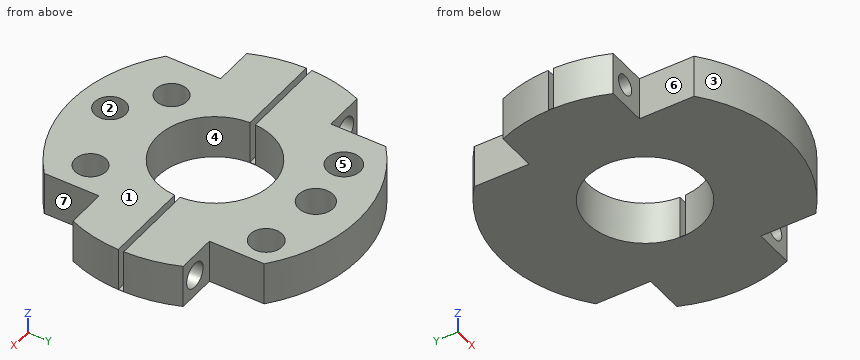
from build123d import *

# Parameters (mm, degrees)
SKETCH_R        = 20
SKETCH_R_2      = 8
PAD_DEPTH       = 6
SKETCH001_R     = 2.4
SKETCH001_R_2   = 2.3
SKETCH001_R_3   = 2.2
SKETCH001_R_4   = 2.15
POCKET_DEPTH    = 4
SKETCH003_W     = 43.022533
SKETCH003_H     = 0.75
POCKET001_DEPTH = 5.95
SKETCH007_W     = 7.6375744751
SKETCH007_H     = 10.86069433
SKETCH007_W_2   = 8.2446434751
SKETCH007_H_2   = 12.05515533
SKETCH007_W_3   = 8.5299164751
SKETCH007_H_3   = 10.94123533
SKETCH007_W_4   = 11.8328734751
SKETCH007_H_4   = 10.66832833
POCKET002_DEPTH = 6.001
SKETCH008_R     = 1.4
POCKET003_DEPTH = 27.65392667
SKETCH009_R     = 1.75
POCKET004_DEPTH = 8


with BuildPart() as part:
    # Sketch → Pad (new body)
    with BuildSketch(Plane.XY):
        Circle(SKETCH_R)
        Circle(SKETCH_R_2, mode=Mode.SUBTRACT)
    extrude(amount=PAD_DEPTH)

    # Sketch001 (on Face4 of Pad) → Pocket (cut)
    with BuildSketch(Plane.XY.offset(6)):
        with Locations((0, 14)):
            Circle(SKETCH001_R)
        with Locations((-7.5, 12.9903810568)):
            Circle(SKETCH001_R_2)
        with Locations((9.1772229816, 13.1064327086)):
            Circle(SKETCH001_R_3)
        with Locations((8.7263178357, -11.5802148957)):
            Circle(SKETCH001_R_4)
        with Locations((-1.3509140126, -15.4410178204)):
            Circle(SKETCH001_R_4)
        with Locations((-7.2695077451, -10.7774884432)):
            Circle(SKETCH001_R_4)
    extrude(amount=-POCKET_DEPTH, mode=Mode.SUBTRACT)

    # Sketch003 (on Face3 of Pocket) → Pocket001 (cut)
    with BuildSketch(Plane.XY.offset(6)):
        with Locations((-0.7364995, 0)):
            Rectangle(SKETCH003_W, SKETCH003_H)
    extrude(amount=-POCKET001_DEPTH, mode=Mode.SUBTRACT)

    # Sketch007 (on Face9 of Pocket001) → Pocket002 (cut, through all)
    with BuildSketch(Plane.XY.offset(6)):
        with Locations((-16.7398847624, -13.083273835)):
            Rectangle(SKETCH007_W, SKETCH007_H)
        with Locations((-17.0434192624, 13.680504335)):
            Rectangle(SKETCH007_W_2, SKETCH007_H_2)
        with Locations((17.1860557624, 13.123544335)):
            Rectangle(SKETCH007_W_3, SKETCH007_H_3)
        with Locations((18.8375342624, -12.987090835)):
            Rectangle(SKETCH007_W_4, SKETCH007_H_4)
    extrude(amount=-POCKET002_DEPTH, mode=Mode.SUBTRACT)

    # Sketch008 → Pocket003 (cut, through all)
    with BuildSketch(Plane(origin=(0, 7.65292667, 0), x_dir=(-1, 0, 0), z_dir=(0, 1, 0))):
        with Locations((-15.963433, 3)):
            Circle(SKETCH008_R)
        with Locations((15.963433, 3)):
            Circle(SKETCH008_R)
    extrude(amount=-POCKET003_DEPTH, mode=Mode.SUBTRACT)

    # Sketch009 → Pocket004 (cut)
    with BuildSketch(Plane(origin=(0, 7.65292667, 0), x_dir=(-1, 0, 0), z_dir=(0, 1, 0))):
        with Locations((-15.997951, 3)):
            Circle(SKETCH009_R)
        with Locations((15.997951, 3)):
            Circle(SKETCH009_R)
    extrude(amount=-POCKET004_DEPTH, mode=Mode.SUBTRACT)


solid = part.part
Input: part model. Units: mm. Frame: model coordinates. Face numbers are marked on the shaded views. A direction names the side the tool comes from. Round coordinates to 2 decimals unless told otherwise and drop trailing zeros. Order: outer loops, then holes, each group sorted by start corner. A loop starts at its lowest first (then second) coordinate and runs counter-clockwise, first axis right, second up. Notation, with made-up numbers: (56.25, 9.5) - (74.25, 9.5) arc R26 ccw to (74.25, 39.5) - close; hole circle Ø4 at (77.25, 74.25). An arc over 180 degrees is marked (long way). Answer as a JSON object with one key per item and string values. Group by question number.
(1) Pin query (flat end, axial travel): P1, Ø1.8, axis at y = 10, z = 2, coming from the +X side; P2, Ø1.3, axis at x = -6.5, y = -10.5, coming from the +Z side; P3, Ø1.7, axis at x = 15, z = 2.5, coming from the +Y side. Return the tip coordinate at first contact, or that it passes through.
(2) Cut plane C-C (x = 15.5). Return loops of the section in (y, z) (3 decimals).
(3) Reachability of the marked faces 5, 6 and 7 from +Z, -Z, +X, -X, +Y, -Y: full face, straight path, thin tool, end or side. Return the list, or none.
(4) Cut plane A-A (y = -7). Return loops of the section in (x, z) (3 decimals).
(5) Draft query along Y for the marked faces 1, 2, 3 and 4. Return one class per face: released by +Y, released by -Y, zero draft, split by the parting line, or undercut.
(6) Cut plane D-D (z = 3). Count the separate pieces of the cut face and the enclosed holes in it, then the cut area to 3 significant figures.
(7) Material intervals for probe 1 along Y at (x, z) = (-13, 2.1) (3 decimals); probe 2 along Y at (x, z) = (-1.5, 3.1); probe 3 along X at (y, z) = (12, 2.9), sorted ascending. Write a range as from..to.
(8) Cut plane B-B (x = -7.5). Return loops of the section in (y, z).
Here are the results:
{
 "1": {"P1": "stops at x = 12.92", "P2": "stops at z = 2", "P3": "stops at y = 7.65"},
 "2": {"outline": "(-7.653, 0) - (7.653, 0) - (7.653, 1.322) - (0.375, 1.322) - (0.375, 0.05) - (-0.375, 0.05) - (-0.375, 1.679) - (-7.653, 1.679) - close; (-7.653, 4.321) - (-0.375, 4.321) - (-0.375, 6) - (-7.653, 6) - close; (0.375, 4.678) - (7.653, 4.678) - (7.653, 6) - (0.375, 6) - close"},
 "3": {"face 5": "+Z", "face 6": "+Z, -Z, -X, -Y", "face 7": "+Z, -Z, +X, -Y"},
 "4": {"outline": "(-18.735, 0) - (-3.873, 0) - (-3.873, 6) - (-18.735, 6) - close; (3.873, 0) - (18.735, 0) - (18.735, 6) - (3.873, 6) - close; hole circle Ø2.8 at (-15.963, 3); hole circle Ø2.8 at (15.963, 3)"},
 "5": {"face 1": "zero draft", "face 2": "undercut", "face 3": "released by -Y", "face 4": "undercut"},
 "6": {"separate pieces": "6", "enclosed holes": "6", "area": "754 mm^2"},
 "7": {"probe 1": "y = -7.653..-0.375, 0.375..7.653", "probe 2": "y = -19.94..-17.59, -13.3..-7.86, 7.86..12.13, 15.87..19.94", "probe 3": "x = -12.92..-9.58, -5.42..-1.33, 1.33..7.28, 11.08..12.92"},
 "8": {"outline": "(-18.54, 0) - (-2.78, 0) - (-2.78, 6) - (-8.64, 6) - (-8.64, 2) - (-12.92, 2) - (-12.92, 6) - (-18.54, 6) - close; (2.78, 0) - (18.54, 0) - (18.54, 6) - (15.29, 6) - (15.29, 2) - (10.69, 2) - (10.69, 6) - (2.78, 6) - close"}
}
